Source: CAD feature listing. Evaluate the final solid. Frame: model axes, mm. A direction names the side the tool comes from. Give positions to 0.01 mm unless a question says otherwise; leave off trailing zeros. Order: outer loops, then holes, each group sorted by start corner. A loop starts at its lowest first (then second) coordinate and runs counter-clockwise, first axis right, second up. Notation, with made-up numbers: M -10.75,61 L 26.25,61 A14 cw 26.25,66 Z; hole C 73.25,40 d6. An arc over 180 degrees is marked long. Answer as a JSON object with one key per item and string values. Group by question number.
1. Section query C-C (y = 20). Output: boundary loops of the cut face in (x, z), plus the area to 3 significant figures.
2. Section query A-A (y = 27.5). Output: boundary loops of the cut face in (x, z), plus the area to 3 significant figures.
3. Pull-direction query (Y, two-part tool) for faces 4 (the cylindrical face through (9.86, 25.492, 9.881)), 5 (the flat face through (10, 15, 10)), 6 (the flat face through (-14, 25, 65)); classes: +Y half, -Y half, draft (parallel to the pull), parting line (faces both ways), or undercut.
4. Pin query (flat end, axial travel): P1, Ø16.5, axis at x = 30, y = 13, coming from the +Z side; P2, Ø8, axis at x = 6, z = 14.5, coming from the -Y side; P3, Ø2, axis at x = 12.5, y = 25, coming from the +Z side. Return the tip coordinate at first contact, or that it passes through.
5. Material intervals for L1, parallel to X at y = 32, z = 69.5; L2, parallel to Y at x = 16, z = 10; L3, parallel to Y at x = 48, z = 75, sorted ascending. Write a range as [from, to].
6. Section query B-B (z = 68). Output: boundary loops of the cut face in (x, y).
7. Set-up query: faces 1 (the flat face through (-29, 20, 85)), 2 (the flat face through (10, 25, 50)), 3 (the flat face through (20, 32, 10)). Return all of +Z, -Z, +X, -X, +Y, -Y with unobstructed straight access to the full face (end or side cutting, diameter ignored); none if empty.
8. Section query D-D (x = 6). Output: boundary loops of the cut face in (y, z), plus the area to 3 significant figures.
from build123d import *

# Parameters (mm, degrees)
BOSS_EXTRUDE2_DEPTH = 50
FILLET3_R           = 10
FILLET4_R           = 10
FILLET5_R           = 5
FILLET6_R           = 5
SKETCH3_W           = 20
SKETCH3_H           = 15
CUT_EXTRUDE2_DEPTH  = 37
SKETCH2_R           = 5
CUT_EXTRUDE3_DEPTH  = 115
CUT_EXTRUDE4_REACH  = 114.432
SKETCH4_R           = 3.3


with BuildPart() as part:
    # Sketch1 → Boss-Extrude2 (new body)
    with BuildSketch(Plane(origin=(0, 0, 0), x_dir=(1, 0, 0), z_dir=(0, 1, 0))):
        Polygon((20, 0), (0, 0), (0, -20), (-34, -20), (-34, -85), (-24, -85), (-24, -65), (1.5, -65), (1.5, -50), (18.5, -50), (18.5, -65), (44, -65), (44, -85), (54, -85), (54, -20), (20, -20), align=None)
    extrude(amount=BOSS_EXTRUDE2_DEPTH)

    # Fillet3
    fillet3_edges = [part.edges().sort_by_distance(p)[0] for p in [
        (-29, 50, 85),
    ]]
    fillet(fillet3_edges, radius=FILLET3_R)

    # Fillet4
    fillet4_edges = [part.edges().sort_by_distance(p)[0] for p in [
        (49, 50, 85),
    ]]
    fillet(fillet4_edges, radius=FILLET4_R)

    # Fillet5
    fillet5_edges = [part.edges().sort_by_distance(p)[0] for p in [
        (1.5, 25, 65),
    ]]
    fillet(fillet5_edges, radius=FILLET5_R)

    # Fillet6
    fillet6_edges = [part.edges().sort_by_distance(p)[0] for p in [
        (18.5, 25, 65),
    ]]
    fillet(fillet6_edges, radius=FILLET6_R)

    # Sketch3 → Cut-Extrude2 (cut)
    with BuildSketch(Plane.ZY):
        with Locations((10, 7.5)):
            Rectangle(SKETCH3_W, SKETCH3_H)
    extrude(amount=-CUT_EXTRUDE2_DEPTH, mode=Mode.SUBTRACT)

    # Sketch2 → Cut-Extrude3 (cut)
    with BuildSketch(Plane.ZY.offset(34)):
        with Locations((75, 20)):
            Circle(SKETCH2_R)
    extrude(amount=-CUT_EXTRUDE3_DEPTH, mode=Mode.SUBTRACT)

    # Sketch4 → Cut-Extrude4 (cut, up to next)
    with BuildSketch(Plane.ZY, mode=Mode.PRIVATE) as cut_extrude4_sk1:
        with Locations((12.5, 42.5)):
            Circle(SKETCH4_R)
    cut_extrude4_tool1 = extrude(cut_extrude4_sk1.sketch, amount=-CUT_EXTRUDE4_REACH, mode=Mode.PRIVATE) & part.part
    # Sketch4 → Cut-Extrude4 (cut, up to next)
    with BuildSketch(Plane.ZY, mode=Mode.PRIVATE) as cut_extrude4_sk2:
        with Locations((12.5, 27.5)):
            Circle(SKETCH4_R)
    cut_extrude4_tool2 = extrude(cut_extrude4_sk2.sketch, amount=-CUT_EXTRUDE4_REACH, mode=Mode.PRIVATE) & part.part
    add(cut_extrude4_tool1.solids().sort_by_distance((0, 42.5, 12.5))[0], mode=Mode.SUBTRACT)
    add(cut_extrude4_tool2.solids().sort_by_distance((0, 27.5, 12.5))[0], mode=Mode.SUBTRACT)


solid = part.part
Answer sheet:
{
 "1": {"outline": "M -34,20 L 0,20 L 0,0 L 20,0 L 20,20 L 54,20 L 54,70 L 44,70 L 44,65 L 23.5,65 A5 ccw 18.5,60 L 18.5,50 L 1.5,50 L 1.5,60 A5 ccw -3.5,65 L -24,65 L -24,70 L -34,70 Z; M -34,80 L -24,80 L -24,85 L -34,85 Z; M 44,80 L 54,80 L 54,85 L 44,85 Z", "area": "4,290 mm^2"},
 "2": {"outline": "M -34,20 L 0,20 L 0,15.8 L 20,15.8 L 20,20 L 54,20 L 54,85 L 44,85 L 44,65 L 23.5,65 A5 ccw 18.5,60 L 18.5,50 L 1.5,50 L 1.5,60 A5 ccw -3.5,65 L -24,65 L -24,85 L -34,85 Z; M 0,0 L 20,0 L 20,9.2 L 0,9.2 Z", "area": "4,360 mm^2"},
 "3": {"face 4": "undercut", "face 5": "-Y half", "face 6": "draft"},
 "4": {"P1": "z = 65", "P2": "y = 15", "P3": "z = 50"},
 "5": {"L1": "[-34, -24], [44, 54]", "L2": "[15, 25.35], [29.65, 40.35], [44.65, 50]", "L3": "[0, 15], [25, 50]"},
 "6": {"outline": "M -34,0 L -24,0 L -24,50 L -34,50 Z; M 44,0 L 54,0 L 54,50 L 44,50 Z"},
 "7": {"face 1": "+Z, +X, -X, +Y, -Y", "face 2": "+Z, +Y, -Y", "face 3": "-Z, +X, +Y, -Y"},
 "8": {"outline": "M 0,20 L 15,20 L 15,0 L 50,0 L 50,50 L 0,50 Z; hole C 27.5,12.5 d6.6; hole C 42.5,12.5 d6.6", "area": "2,130 mm^2"}
}
